from build123d import *

# Parameters (mm, degrees)
EXTRUDE_THIN1_DEPTH       = 60
SKETCH2_R                 = 3
CUT_EXTRUDE1_DEPTH        = 10
LPATTERN1_COUNT           = 2
LPATTERN1_PITCH           = 30
LPATTERN2_COUNT           = 2
LPATTERN2_PITCH           = 150
LPATTERN2_COPY_1_SKETCH_R = 3
LPATTERN2_COPY_1_DEPTH    = 10
FILLET1_R                 = 10
FILLET2_R                 = 10
FILLET3_R                 = 5
FILLET4_R                 = 5


with BuildPart() as part:
    # Sketch1 → Extrude-Thin1 (new body)
    with BuildSketch(Plane.XY):
        Polygon((30, -56.94), (0, -56.94), (0, 0), (-120.8, 0), (-120.8, -56.94), (-150.8, -56.94), (-150.8, -59.94), (-117.8, -59.94), (-117.8, -3), (-3, -3), (-3, -59.94), (30, -59.94), align=None)
    extrude(amount=EXTRUDE_THIN1_DEPTH)

    # Sketch2 → Cut-Extrude1 (cut)
    with BuildSketch(Plane(origin=(0, -56.94, 0), x_dir=(1, 0, 0), z_dir=(0, 1, 0))):
        with Locations(Location((15, -15, 0), (0, 0, 270))):
            Circle(SKETCH2_R)
    cut_extrude1 = extrude(amount=-CUT_EXTRUDE1_DEPTH, mode=Mode.SUBTRACT)

    # LPattern1: Cut-Extrude1 ×2
    with Locations(*[(0, 0, i * LPATTERN1_PITCH) for i in range(1, LPATTERN1_COUNT)]):
        add(cut_extrude1, mode=Mode.SUBTRACT)

    # LPattern2: Cut-Extrude1 ×2
    with Locations(*[(-i * LPATTERN2_PITCH, 0, 0) for i in range(1, LPATTERN2_COUNT)]):
        add(cut_extrude1, mode=Mode.SUBTRACT)

    # LPattern2 copy 1 sketch → LPattern2 copy 1 (cut)
    with BuildSketch(Plane(origin=(-150, -56.94, 30), x_dir=(1, 0, 0), z_dir=(0, 1, 0))):
        with Locations(Location((15, -15, 0), (0, 0, 270))):
            Circle(LPATTERN2_COPY_1_SKETCH_R)
    extrude(amount=-LPATTERN2_COPY_1_DEPTH, mode=Mode.SUBTRACT)

    # Fillet1
    fillet1_edges = [part.edges().sort_by_distance(p)[0] for p in [
        (-120.8, 0, 30),
        (0, 0, 30),
    ]]
    fillet(fillet1_edges, radius=FILLET1_R)

    # Fillet2
    fillet2_edges = [part.edges().sort_by_distance(p)[0] for p in [
        (-3, -3, 30),
        (-117.8, -3, 30),
    ]]
    fillet(fillet2_edges, radius=FILLET2_R)

    # Fillet3
    fillet3_edges = [part.edges().sort_by_distance(p)[0] for p in [
        (-120.8, -56.94, 30),
        (0, -56.94, 30),
    ]]
    fillet(fillet3_edges, radius=FILLET3_R)

    # Fillet4
    fillet4_edges = [part.edges().sort_by_distance(p)[0] for p in [
        (-3, -59.94, 30),
        (-117.8, -59.94, 30),
    ]]
    fillet(fillet4_edges, radius=FILLET4_R)


solid = part.part
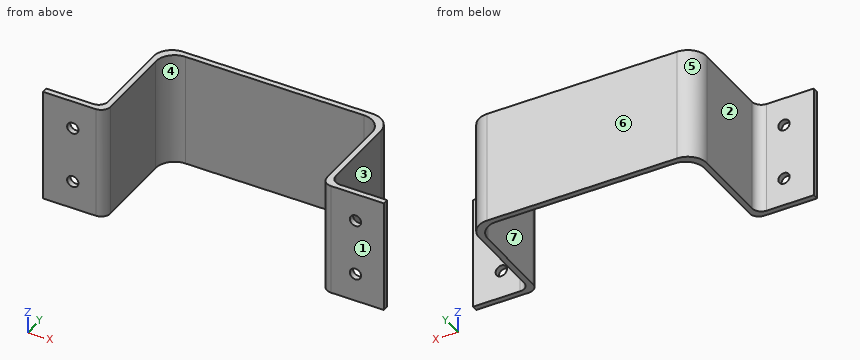
Here's how the part is built. I have some questions about the finished solid (model axes, mm). Face numbers are marked on the shaded views. A direction names the side the tool comes from. Round coordinates to 2 decimals unless told otherwise and drop trailing zeros. Write each loop counter-clockwise with the first axis right and the second up, starting at its lowest first coordinate (ties: lowest second). Pieces come first, ordered by that corner, then holes.
1. I need wall thicknesses on L1, parallel to Z at x = -135, y = -58; L2, parallel to X at y = -35.5, z = 7; L3, parallel to X at y = -59, z = 45. Which ranges of each line are inside material? Lowest first, please.
2. Suppose I cut it at A-A (z = 45). List the corners of the cut face in (x, y) for me.
3. If we mould it in two halves opening along X, with no side actions, what happens to the marked faces 5, 6 and 7? For each: released by +X, released by -X, zero draft, split by the parting line, or undercut.
4. Suppose I cut it at C-C (x = 15). List the corners of the cut face in (y, z) for me, and give its area (3 significant figures).
5. Suppose I cut it at B-B (y = -39). List the corners of the cut face in (x, z) for me, and give its area (3 significant figures).
6. Suppose I cut it at D-D (z = 31). List the corners of the cut face in (x, y) for me, and give its area (3 significant figures).
7. For the marked faces 1, 2, 3 and 4, which set-ups out of +Z, -Z, +X, -X, +Y, -Y let a thin tool reach every point of the face, with its end or its side?
8. Will these pins go through, and if not, where does the flat tip stop? pin 1 Ø6 at (y, z) = (-34.5, 41.5) entering from +X; pin 2 Ø3 at (x, z) = (-3, 40.5) entering from -Y; pin 3 Ø20 at (x, z) = (23, 34) entering from +Y.
Answer sheet:
1. L1: z = 0 to 12, 18 to 42, 48 to 60
1. L2: x = -120.8 to -117.8, -3 to 0
1. L3: x = -150.8 to -138, -132 to -119.88, -0.92 to 12, 18 to 30
2. outline: (-150.8, -59.94) - (-138, -59.94) - (-138, -56.94) - (-150.8, -56.94) - close; (-132, -59.94) - (-122.8, -59.94) arc R5 ccw to (-117.8, -54.94) - (-117.8, -13) arc R10 cw to (-107.8, -3) - (-13, -3) arc R10 cw to (-3, -13) - (-3, -54.94) arc R5 ccw to (2, -59.94) - (12, -59.94) - (12, -56.94) - (5, -56.94) arc R5 cw to (0, -51.94) - (0, -10) arc R10 ccw to (-10, 0) - (-110.8, 0) arc R10 ccw to (-120.8, -10) - (-120.8, -51.94) arc R5 cw to (-125.8, -56.94) - (-132, -56.94) - close; (18, -59.94) - (30, -59.94) - (30, -56.94) - (18, -56.94) - close
3. face 5: released by -X
3. face 6: zero draft
3. face 7: undercut
4. outline: (-59.94, 0) - (-56.94, 0) - (-56.94, 12) - (-59.94, 12) - close; (-59.94, 18) - (-56.94, 18) - (-56.94, 42) - (-59.94, 42) - close; (-59.94, 48) - (-56.94, 48) - (-56.94, 60) - (-59.94, 60) - close
4. area: 144 mm2
5. outline: (-120.8, 0) - (-117.8, 0) - (-117.8, 60) - (-120.8, 60) - close; (-3, 0) - (0, 0) - (0, 60) - (-3, 60) - close
5. area: 360 mm2
6. outline: (-150.8, -59.94) - (-122.8, -59.94) arc R5 ccw to (-117.8, -54.94) - (-117.8, -13) arc R10 cw to (-107.8, -3) - (-13, -3) arc R10 cw to (-3, -13) - (-3, -54.94) arc R5 ccw to (2, -59.94) - (30, -59.94) - (30, -56.94) - (5, -56.94) arc R5 cw to (0, -51.94) - (0, -10) arc R10 ccw to (-10, 0) - (-110.8, 0) arc R10 ccw to (-120.8, -10) - (-120.8, -51.94) arc R5 cw to (-125.8, -56.94) - (-150.8, -56.94) - close
6. area: 884 mm2
7. face 1: +Z, -Z, +X, -X, -Y
7. face 2: +Z, -Z, -X, +Y
7. face 3: +Z, -Z, +X, +Y
7. face 4: +Z, -Z, -Y
8. pin 1: stops at x = 0
8. pin 2: stops at y = -58.51
8. pin 3: stops at y = -56.94
